Part model, mm, in its own coordinate system. A direction names the side the tool comes from. Coordinates: 2 decimals unless noted, no trailing zeros. Write each loop counter-clockwise with the first axis right and the second up, starting at its lowest first coordinate (ties: lowest second). Pieces come first, ordered by that corner, then holes. Notation, with made-up numbers: M -14.5,21.5 L 34.5,21.5 A14 cw 34.5,42.5 Z; hole C 58.5,12 d11. An arc over 180 degrees is marked long. Use a Markdown table: item, result. Add a question column.
Q1. Slice it at D-D on x = -21. Write the cut outline in (y, z).
Q2. Wall check: L1, parallel to Y at x = -1, z = 3.25; L2, parallel to Y at x = -22.5, z = -8.2. Give the ranges that are in metal, low to high. Write a range as from..to.
Q3. Slice it at C-C on y = 0. Count the separate pieces of the cut face and the enclosed holes in it, then the cut area to 3 significant figures.
Q4. Slice it at A-A on z = 4.5. Write the cut outline in (x, y), then the cut area to 3 significant figures.
Q5. Slice it at B-B on x = 17. Write the cut outline in (y, z).
Q6. Tool access for faces 1 (the conical face through (-31.7, -0.2, 7.2)), 2 (the flat face through (12.5, 8, 0)), 3 (the cylindrical face through (25, 0, -8)), 4 (the flat face through (-12.5, -8, 0)), 5 (the conical face through (31.7, -0.2, 7.2)): list every direction of +Z, -Z, +X, -X, +Y, -Y with a clear straight run to the whole face (end or side of a thin tool).
Q7. Pin check, flat tips, straight feed: pin 1 Ø4 at (x, y) = (-22.5, 0) entering from -Z; pin 2 Ø1.6 at (y, z) = (7.5, 1.5) entering from +X; pin 3 Ø1.6 at (y, z) = (-8.5, -1.5) entering from -X; pin 4 Ø8 at (y, z) = (7, 5) entering from -X. Stop position of each tip, or through.
Q8. Mould opens along Z. For faces 6 (the conical face through (-31.7, -0.2, -9.8)), 7 (the flat face through (0, 7, 0)), 8 (the cylindrical face through (-25, 0, 8)) say: released by +Z, released by -Z, zero draft, split by the parting line, or undercut.
from build123d import *

# Parameters (mm, degrees)
BOSS_EXTRUDE1_DEPTH = 10
CUT_EXTRUDE1_DEPTH  = 7
SKETCH3_R           = 2.5
CUT_EXTRUDE2_DEPTH  = 10
CHAMFER2_SIZE       = 1
CHAMFER3_SIZE       = 1
SHELL1_START        = -7
SHELL1_OUTLINE_W    = 25
SHELL1_OUTLINE_H    = 14
SHELL1_DEPTH        = 14
CHAMFER4_SIZE       = 1


# Read off the part's stored shape, not the designer's step: Shell1
with BuildPart() as part:
    # Sketch1 → Boss-Extrude1 (new, symmetric)
    with BuildSketch(Plane.XY):
        with BuildLine():
            Line((-22.5, 10), (22.5, 10))
            ThreePointArc((22.5, 10), (32.5, 0), (22.5, -10))
            Line((22.5, -10), (-22.5, -10))
            ThreePointArc((-22.5, -10), (-32.5, 0), (-22.5, 10))
        make_face()
    extrude(amount=BOSS_EXTRUDE1_DEPTH, both=True)

    # Sketch2 → Cut-Extrude1 (cut, symmetric)
    with BuildSketch(Plane.XY):
        with BuildLine():
            Line((-22.5, 10), (-12.5, 10))
            Line((-12.5, 10), (-12.5, -10))
            Line((-12.5, -10), (-22.5, -10))
            ThreePointArc((-22.5, -10), (-32.5, 0), (-22.5, 10))
        make_face()
        with BuildLine():
            Line((12.5, -10), (22.5, -10))
            ThreePointArc((22.5, -10), (32.5, 0), (22.5, 10))
            Line((22.5, 10), (12.5, 10))
            Line((12.5, 10), (12.5, -10))
        make_face()
    extrude(amount=CUT_EXTRUDE1_DEPTH, both=True, mode=Mode.SUBTRACT)

    # Sketch3 → Cut-Extrude2 (cut, symmetric)
    with BuildSketch(Plane.XY):
        with Locations((-22.5, 0)):
            Circle(SKETCH3_R)
        with Locations(Location((22.5, 0, 0), (0, 0, 180))):
            Circle(SKETCH3_R)
    extrude(amount=CUT_EXTRUDE2_DEPTH, both=True, mode=Mode.SUBTRACT)

    # Chamfer2
    chamfer2_edges = [part.edges().sort_by_distance(p)[0] for p in [
        (-32.5, 0, -7),
        (-17.5, 10, -7),
        (-17.5, -10, -7),
        (-32.5, 0, 7),
        (-17.5, -10, 7),
        (-17.5, 10, 7),
        (32.5, 0, -7),
        (17.5, -10, -7),
        (17.5, 10, -7),
        (32.5, 0, 7),
        (17.5, 10, 7),
        (17.5, -10, 7),
    ]]
    chamfer(chamfer2_edges, length=CHAMFER2_SIZE)

    # Chamfer3
    chamfer3_edges = [part.edges().sort_by_distance(p)[0] for p in [
        (32.5, 0, 10),
        (0, 10, 10),
        (-32.5, 0, 10),
        (0, 10, -10),
        (32.5, 0, -10),
        (0, -10, -10),
        (-32.5, 0, -10),
        (0, -10, 10),
    ]]
    chamfer(chamfer3_edges, length=CHAMFER3_SIZE)

    # Shell1 outline → Shell1 (cut)
    with BuildSketch(Plane.XY.offset(SHELL1_START)):
        Rectangle(SHELL1_OUTLINE_W, SHELL1_OUTLINE_H)
    extrude(amount=SHELL1_DEPTH, mode=Mode.SUBTRACT)

    # Chamfer4
    chamfer4_edges = [part.edges().sort_by_distance(p)[0] for p in [
        (12.5, -10, 0),
        (12.5, 10, 0),
        (-12.5, -10, 0),
        (-12.5, 10, 0),
    ]]
    chamfer(chamfer4_edges, length=CHAMFER4_SIZE)


solid = part.part
Recorded:
| question | item | result |
|---|---|---|
| 1 | outline | M -10,-9 L -9,-10 L -2,-10 L -2,-7 L -9,-7 L -10,-8 Z; M -10,8 L -9,7 L -2,7 L -2,10 L -9,10 L -10,9 Z; M 2,-10 L 9,-10 L 10,-9 L 10,-8 L 9,-7 L 2,-7 Z; M 2,7 L 9,7 L 10,8 L 10,9 L 9,10 L 2,10 Z |
| 2 | L1 | -10..-7, 7..10 |
| 2 | L2 | -10..-2.5, 2.5..10 |
| 3 | separate pieces | 6 |
| 3 | enclosed holes | 0 |
| 3 | area | 326 mm² |
| 4 | outline | M -12.5,-9 L -11.5,-10 L 11.5,-10 L 12.5,-9 L 12.5,-7 L -12.5,-7 Z; M -12.5,7 L 12.5,7 L 12.5,9 L 11.5,10 L -11.5,10 L -12.5,9 Z |
| 4 | area | 148 mm² |
| 5 | outline | M -10,-9 L -9,-10 L 9,-10 L 10,-9 L 10,-8 L 9,-7 L -9,-7 L -10,-8 Z; M -10,8 L -9,7 L 9,7 L 10,8 L 10,9 L 9,10 L -9,10 L -10,9 Z |
| 6 | face 1 | -X |
| 6 | face 2 | +X, +Y, -Y |
| 6 | face 3 | +Z, -Z |
| 6 | face 4 | -X, +Y, -Y |
| 6 | face 5 | +X |
| 7 | pin 1 | through |
| 7 | pin 2 | x = 12.5 |
| 7 | pin 3 | x = -12.5 |
| 7 | pin 4 | x = -31.5 |
| 8 | face 6 | released by -Z |
| 8 | face 7 | undercut |
| 8 | face 8 | zero draft |
